Geometry check sheet. Reference: the model listing, model coordinates, mm. A direction names the side the tool comes from. Round coordinates to 2 decimals unless told otherwise and drop trailing zeros. Order: outer loops, then holes, each group sorted by start corner. A loop starts at its lowest first (then second) coordinate and runs counter-clockwise, first axis right, second up. Notation, with made-up numbers: (51.25, 60.25) - (106.25, 60.25) arc R37 ccw to (106.25, 98.25) - close; hole circle Ø5 at (43.25, 64.25). An arc over 180 degrees is marked (long way). Return JSON: item names as keys, results as strings. Group by question number.
Q1. Tool access check on faces 4 (the flat face through (-3, 3, 195.396)), 5 (the flat face through (-6.628, 3, 54)). Record the directions out of +Z, -Z, +X, -X, +Y, -Y that give a thin tool (end or side, any length) a straight path to the whole face; none if there is none.
Q2. Draft check along Z on faces 1 (the flat face through (-3, 3, -14.604)), 2 (the flat face through (-3, 6, 112)), 3 (the flat face through (-3, 3, 58.396)). Enter one of: pulls with the +Z half, pulls with the -Z half, needs draft (parallel to the pull), parting line crosses it, or undercut.
Q3. Sectioned sample at A-A, the plane y = 4.2. Record the cut outline in (x, z), then the cut area to 3 significant figures.
Q4. Material ranges on line 1 along Z through (x, y) = (4.25, 4.6); line 2 along Z through (x, y) = (-3.5, 5.2); line 3 along Z through (x, y) = (1.5, 4.35), recorded low to high.
```python
from build123d import *

# Parameters (mm, degrees)
SKETCH_1_W          = 25
SKETCH_1_H          = 210
EXTRUDE_1_DEPTH     = 6
SKETCH_2_R          = 1.55
CUT_EXTRUDE_1_DEPTH = 6
SKETCH_3_R          = 1.25
CUT_EXTRUDE_2_DEPTH = 6


with BuildPart() as part:
    # Эскиз1 → Бобышка-Вытянуть1 (new body)
    with BuildSketch(Plane(origin=(0, 0, 0), x_dir=(1, 0, 0), z_dir=(0, 1, 0))):
        with Locations((-3.127715508, -90.396451994)):
            Rectangle(SKETCH_1_W, SKETCH_1_H)
    extrude(amount=EXTRUDE_1_DEPTH)

    # Эскиз2 → Вырез-Вытянуть1 (cut)
    with BuildSketch(Plane(origin=(0, 6, 0), x_dir=(1, 0, 0), z_dir=(0, 1, 0))):
        with Locations(Location((-3.127715508, 4.603548006, 0), (0, 0, 270))):
            Circle(SKETCH_2_R)
        with Locations(Location((-3.127715508, -185.396451994, 0), (0, 0, 90))):
            Circle(SKETCH_2_R)
    extrude(amount=-CUT_EXTRUDE_1_DEPTH, mode=Mode.SUBTRACT)

    # Эскиз3 → Вырез-Вытянуть2 (cut)
    with BuildSketch(Plane(origin=(0, 6, 0), x_dir=(1, 0, 0), z_dir=(0, 1, 0))):
        with Locations(Location((-8.127715508, -54.396451994, 0), (0, 0, 270))):
            Circle(SKETCH_3_R)
        with Locations(Location((1.872284492, -54.396451994, 0), (0, 0, 90))):
            Circle(SKETCH_3_R)
        with Locations(Location((1.872284492, -6.396451994, 0), (0, 0, 270))):
            Circle(SKETCH_3_R)
        with Locations(Location((-8.127715508, -6.396451994, 0), (0, 0, 90))):
            Circle(SKETCH_3_R)
        Polygon((-13.127715508, -10.396451994), (6.872284492, -10.396451994), (6.872284492, -50.396451994), (0.372284492, -50.396451994), (0.372284492, -58.396451994), (-6.627715508, -58.396451994), (-6.627715508, -50.396451994), (-13.127715508, -50.396451994), align=None)
    extrude(amount=-CUT_EXTRUDE_2_DEPTH, mode=Mode.SUBTRACT)


solid = part.part
```
Reply:
{
 "1": {"face 4": "+Z, +X, -X, +Y, -Y", "face 5": "+Y, -Y"},
 "2": {"face 1": "pulls with the -Z half", "face 2": "needs draft", "face 3": "undercut"},
 "3": {"outline": "(-15.63, -14.6) - (9.37, -14.6) - (9.37, 195.4) - (-15.63, 195.4) - close; hole (-13.13, 10.4) - (6.87, 10.4) - (6.87, 50.4) - (0.37, 50.4) - (0.37, 58.4) - (-6.63, 58.4) - (-6.63, 50.4) - (-13.13, 50.4) - close; hole circle Ø2.5 at (-8.13, 6.4); hole circle Ø2.5 at (-8.13, 54.4); hole circle Ø3.1 at (-3.13, -4.6); hole circle Ø3.1 at (-3.13, 185.4); hole circle Ø2.5 at (1.87, 6.4); hole circle Ø2.5 at (1.87, 54.4)", "area": "4,360 mm^2"},
 "4": {"line 1": "-14.6 to 10.4, 50.4 to 195.4", "line 2": "-14.6 to -6.11, -3.1 to 10.4, 58.4 to 183.89, 186.9 to 195.4", "line 3": "-14.6 to 5.2, 7.59 to 10.4, 50.4 to 53.2, 55.59 to 195.4"}
}
